Verification items for the finished model (mm, model axes). A direction names the side the tool comes from. Coordinates: 2 decimals unless noted, no trailing zeros. Write each loop counter-clockwise with the first axis right and the second up, starting at its lowest first coordinate (ties: lowest second). Pieces come first, ordered by that corner, then holes. Notation, with made-up numbers: (19, -20) -> (52, -20) arc R17 ccw to (52, 5) -> close; hole circle Ø4 at (-37.75, -30.75). An arc over 180 degrees is marked (long way). Write each question's results on one line, items separated by ' | '. Start each with the question number.
from build123d import *

# Parameters (mm, degrees)
ESQUISSE1_W             = 61.168999858
ESQUISSE1_H             = 44.751998484
ESQUISSE1_R             = 3.815511502
BOSS_EXTRU_2_DEPTH      = 4
BOSS_EXTRU_4_START      = 4
ESQUISSE2_R             = 11.783463465
BOSS_EXTRU_4_DEPTH      = 6
ENL_V_MAT_EXTRU_1_DEPTH = 4
ESQUISSE1_2_R           = 3.815511502
ENL_V_MAT_EXTRU_3_DEPTH = 40.193073087
SKETCH1_R               = 1.65
CUT_EXTRUDE1_DEPTH      = 10


with BuildPart() as part:
    # Esquisse1 → Boss.-Extru.2 (new body)
    with BuildSketch(Plane.XY):
        Rectangle(ESQUISSE1_W, ESQUISSE1_H)
        Circle(ESQUISSE1_R, mode=Mode.SUBTRACT)
    extrude(amount=BOSS_EXTRU_2_DEPTH)

    # Esquisse2 → Boss.-Extru.4 (add)
    with BuildSketch(Plane.XY.offset(BOSS_EXTRU_4_START)):
        with Locations(Location((0, 0, 0), (0, 0, 180))):
            Circle(ESQUISSE2_R)
    extrude(amount=BOSS_EXTRU_4_DEPTH)

    # Esquisse4 → Enl_v. mat.-Extru.1 (cut)
    with BuildSketch(Plane.XY.offset(10)):
        with BuildLine():
            Line((2.87019869, 2.302904251), (2.212319523, 10.306766943))
            ThreePointArc((2.212319523, 10.306766943), (-0.029730087, 11.070975118), (-2.223029733, 10.17641531))
            Line((-2.223029733, 10.17641531), (-2.870198645, 2.302904307))
            ThreePointArc((-2.870198645, 2.302904307), (-3.679865285, 0), (-2.870198645, -2.302904307))
            Line((-2.870198645, -2.302904307), (-2.223029733, -10.17641531))
            ThreePointArc((-2.223029733, -10.17641531), (-0.029730087, -11.070975118), (2.212319523, -10.306766943))
            Line((2.212319523, -10.306766943), (2.87019869, -2.302904251))
            ThreePointArc((2.87019869, -2.302904251), (3.679865285, 0), (2.87019869, 2.302904251))
        make_face()
    extrude(amount=-ENL_V_MAT_EXTRU_1_DEPTH, mode=Mode.SUBTRACT)

    # Esquisse1_2 → Enl_v. mat.-Extru.3 (cut, through all)
    with BuildSketch(Plane.XY):
        with Locations(Location((0, 0, 0), (0, 0, 138.351064991))):
            Circle(ESQUISSE1_2_R)
    extrude(amount=ENL_V_MAT_EXTRU_3_DEPTH, mode=Mode.SUBTRACT)

    # Sketch1 → Cut-Extrude1 (cut)
    with BuildSketch(Plane.XY.offset(4)):
        with Locations((-25.584499929, 17.375999242)):
            Circle(SKETCH1_R)
        with Locations(Location((25.584499929, 17.375999242, 0), (0, 0, 180))):
            Circle(SKETCH1_R)
        with Locations((25.584499929, -17.375999242)):
            Circle(SKETCH1_R)
        with Locations(Location((-25.584499929, -17.375999242, 0), (0, 0, 180))):
            Circle(SKETCH1_R)
    extrude(amount=-CUT_EXTRUDE1_DEPTH, mode=Mode.SUBTRACT)


solid = part.part
1. Tool access check on faces 4 (the flat face through (-2.54, -6.3, 8.03)), 5 (the flat face through (30.584, 0, 2)). Record the directions out of +Z, -Z, +X, -X, +Y, -Y that give a thin tool (end or side, any length) a straight path to the whole face; none if there is none.
2. Sectioned sample at B-B on y = 7. Record the cut outline in (x, z), plus the area to 3 significant figures.
3. Depth check by flat-ended pin: pin 1 Ø4.5 at (x, y) = (0, 6.5) entering from +Z; pin 2 Ø12 at (x, y) = (-20.5, -6.5) entering from +Z; pin 3 Ø3 at (y, z) = (12, 7.5) entering from -X. Enter the tip coordinate at first touch or a pass-through.
4. Material ranges on probe 1 along Z at (x, y) = (-11, -17.5); probe 2 along Z at (x, y) = (-2, 8.5); probe 3 along Y at (x, z) = (1, 3.75), recorded low to high. Write a range as from..to.
5. Sectioned sample at A-A on x = 8. Record the cut outline in (y, z).
6. Mould release check, pull along X, two halves, no side actions. Record for faces 1 (the cylindrical face through (9.35, 7.17, 6.96)), 2 (the flat face through (2.527, -6.476, 8.028)), 3 (the flat face through (-7, 10, 4)): +X half, -X half, draft (parallel to the pull), parting line (faces both ways), or undercut.
7. Sectioned sample at C-C on x = -22.5. Record the cut outline in (y, z), plus the area to 3 significant figures.
Computed values:
1) face 4: +Z | face 5: +Z, -Z, +X, +Y, -Y
2) outline: (-30.58, 0) -> (30.58, 0) -> (30.58, 4) -> (9.48, 4) -> (9.48, 10) -> (2.48, 10) -> (2.48, 6) -> (-2.48, 6) -> (-2.48, 10) -> (-9.48, 10) -> (-9.48, 4) -> (-30.58, 4) -> close | area: 339 mm^2
3) pin 1: stops at z = 6 | pin 2: stops at z = 4 | pin 3: stops at x = -5.35
4) probe 1: z = 0..4 | probe 2: z = 0..6 | probe 3: y = -22.38..-3.68, 3.68..22.38
5) outline: (-22.38, 0) -> (22.38, 0) -> (22.38, 4) -> (8.65, 4) -> (8.65, 10) -> (-8.65, 10) -> (-8.65, 4) -> (-22.38, 4) -> close
6) face 1: parting line | face 2: undercut | face 3: draft
7) outline: (-22.38, 0) -> (22.38, 0) -> (22.38, 4) -> (-22.38, 4) -> close | area: 179 mm^2
